Could you check a few things on this model? Use its own coordinates, in mm. A direction names the side the tool comes from. Round coordinates to 2 decimals unless told otherwise and drop trailing zeros. Loops run counter-clockwise (first coordinate to the right, second up) from the corner with the lowest first, then second, coordinate; pieces in that order, holes last. Notation, with made-up numbers: (-6.75, 41) - (19.25, 41) arc R19 cw to (19.25, 45) - close; hole circle Ø11 at (-38, 73). An arc over 180 degrees is marked (long way). Use one line per item in the form item = value.
```python
from build123d import *

# Parameters (mm, degrees)
EXTRUDE_1_DEPTH     = 37
CUT_EXTRUDE_1_DEPTH = 3


with BuildPart() as part:
    # Эскиз1 → Бобышка-Вытянуть1 (new body)
    with BuildSketch(Plane.XY):
        with BuildLine():
            Line((-3, 6.873863542), (-3, 10.583005244))
            ThreePointArc((-3, 10.583005244), (0, -11), (3, 10.583005244))
            Line((3, 10.583005244), (3, 6.873863542))
            ThreePointArc((3, 6.873863542), (0, -7.5), (-3, 6.873863542))
        make_face()
    extrude(amount=-EXTRUDE_1_DEPTH)

    # Эскиз2 → Вырез-Вытянуть1 (cut)
    with BuildSketch(Plane(origin=(0, -11, 0), x_dir=(-1, 0, 0), z_dir=(0, -1, 0))):
        with BuildLine():
            Line((3, 31), (3, 6))
            ThreePointArc((3, 6), (0, 3), (-3, 6))
            Line((-3, 6), (-3, 31))
            ThreePointArc((-3, 31), (0, 34), (3, 31))
        make_face()
    extrude(amount=-CUT_EXTRUDE_1_DEPTH, mode=Mode.SUBTRACT)


solid = part.part
```
1. On a 3-axis mill with a long thin cutter (end or side, diameter ignored), from which of +Z, -Z, +X, -X, +Y, -Y can I reach the whole of each face in a straight line? I mean faces 4 (the face through (2.3, -7.3, 0)), 5 (the face through (0, -10, -34)), 6 (the face through (-3, 9, -18)). Say none if no direction works.
Solution:
face_4 = +Z, +X, -X, +Y, -Y
face_5 = -Y
face_6 = +Z, -Z, +Y
2. If we section it at A-A, the plane y = 0: Write out the boundary of the cut face in (x, z).
Solution:
outline = (-11, -37) - (-7.5, -37) - (-7.5, 0) - (-11, 0) - close; (7.5, -37) - (11, -37) - (11, 0) - (7.5, 0) - close
3. If we section it at D-D, the plane x = 0: Write out the boundary of the cut face in (y, z), plus the area to 3 significant figures.
Solution:
outline = (-11, -37) - (-7.5, -37) - (-7.5, 0) - (-11, 0) - (-11, -3) - (-8, -3) - (-8, -34) - (-11, -34) - close
area = 36.5 mm^2
4. If we section it at C-C, the plane z = -26: Write out the boundary of the cut face in (x, y), plus the area to 3 significant figures.
Solution:
outline = (-3, -10.58) - (-3, -8) - (3, -8) - (3, -10.58) arc R11 ccw to (3, 10.58) - (3, 6.87) arc R7.5 cw (long way) to (-3, 6.87) - (-3, 10.58) arc R11 ccw to start
area = 165 mm^2
5. If we section it at B-B, the plane x = 4.5: Write out the boundary of the cut face in (y, z).
Solution:
outline = (-10.04, -37) - (-6, -37) - (-6, 0) - (-10.04, 0) - close; (6, -37) - (10.04, -37) - (10.04, 0) - (6, 0) - close
6. Please list where these lines run through material, in increasing order: line 1 along X through (y, z) = (0, -9); line 2 along Y through (x, z) = (0, -15.5); line 3 along X through (y, z) = (-5.25, -30.5).
Solution:
line_1 = -11 to -7.5, 7.5 to 11
line_2 = -8 to -7.5
line_3 = -9.67 to -5.36, 5.36 to 9.67
7. For P1, Ø1.5, axis at y = -5, z = -12, coming from the +X side; P2, Ø1.1, axis at y = 8.5, z = -12, coming from the +X side; P3, Ø4, axis at y = 8, z = -12, coming from the -X side, each with a flat end and sliding along its axis, tell me the tip position at first contact or that it passes through.
Solution:
P1 = 10.15
P2 = 7.6
P3 = -9.22
8. We'd pull the mould along X, two halves only. Please class faces 1 (the face through (2.3, -7.3, -37)), 2 (the face through (-6.89, -8.575, -18.241)), 3 (the face through (0.287, -7.495, -18.241)): +X half, -X half, draft (parallel to the pull), parting line (faces both ways), or undercut.
Solution:
face_1 = draft
face_2 = parting line
face_3 = undercut
